Part print with two shaded views. Sizes in mm from the minimum x, y, z corner. A direction names the side the tool comes from. Round coordinates to 2 decimals unless told otherwise and drop trailing zeros. Order: outer loops, then holes, each group sorted by start corner. A loop starts at its lowest first (then second) coordinate and runs counter-clockwise, first axis right, second up. Notation, with made-up numbers: (85, 15.25) -> (133, 15.25) arc R13 ccw to (133, 29.25) -> close; hole circle Ø8 at (-14.5, 45.5). An arc over 180 degrees is marked (long way). Answer as a JSON object with one key per item and string values.
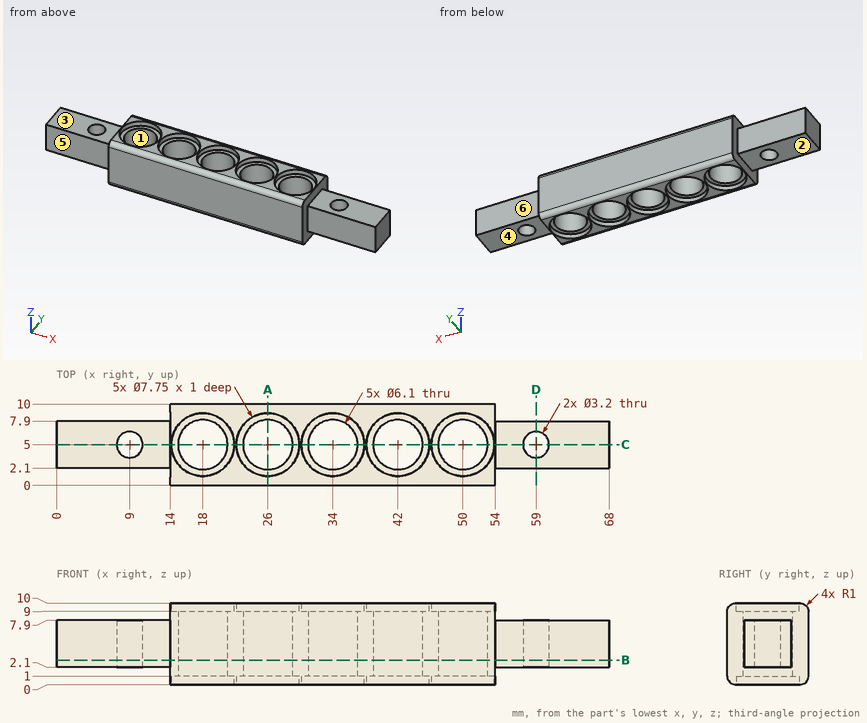
1) Cut at B-B, the plane z = 3. Give the cut face in (x, y), plus the area to 3 significant figures.
Checked values:
{"outline": "(0, 2.1) -> (14, 2.1) -> (14, 0) -> (54, 0) -> (54, 2.1) -> (68, 2.1) -> (68, 7.9) -> (54, 7.9) -> (54, 10) -> (14, 10) -> (14, 7.9) -> (0, 7.9) -> close; hole circle Ø3.2 at (9, 5); hole circle Ø6.1 at (18, 5); hole circle Ø6.1 at (26, 5); hole circle Ø6.1 at (34, 5); hole circle Ø6.1 at (42, 5); hole circle Ø6.1 at (50, 5); hole circle Ø3.2 at (59, 5)", "area": "400 mm²"}
2) Pull direction X, two halves, no side cores. Call the marked faces 1 and 2: pulls with the +X half, pulls with the -X half, needs draft (parallel to the pull), parting line crosses it, or undercut.
Checked values:
{"face 1": "undercut", "face 2": "needs draft"}
3) Cut at A-A, the plane x = 26. Give the cut face in (y, z) (3 decimals).
Checked values:
{"outline": "(0, 1) arc R1 ccw to (1, 0) -> (1.125, 0) -> (1.125, 1) -> (1.95, 1) -> (1.95, 9) -> (1.125, 9) -> (1.125, 10) -> (1, 10) arc R1 ccw to (0, 9) -> close; (8.05, 1) -> (8.875, 1) -> (8.875, 0) -> (9, 0) arc R1 ccw to (10, 1) -> (10, 9) arc R1 ccw to (9, 10) -> (8.875, 10) -> (8.875, 9) -> (8.05, 9) -> close"}
4) Flat gauge pins, fed straight in: pin 1 Ø2.5 at (x, y) = (43, 6) entering from +Z; pin 2 Ø1 at (y, z) = (7, 1.5) entering from +X; pin 3 Ø4.5 at (x, z) = (64.5, 5.5) entering from +Y; pin 4 Ø1.5 at (x, y) = (49, 2.5) entering from -Z. Where does each tip first touch, or does it go through?
Checked values:
{"pin 1": "passes through", "pin 2": "stops at x = 54", "pin 3": "stops at y = 7.9", "pin 4": "stops at z = 1"}
5) Probe L1, parallel to X at y = 6.5, z = 2; L2, parallel to X at y = 7.75, z = 2; L3, parallel to Y at x = 30.5, z = 0.5. List the from-to ranges inside material, lowest first. Write a range as from..to.
Checked values:
{"L1": "x = 14..15.34, 20.66..23.34, 28.66..31.34, 36.66..39.34, 44.66..47.34, 52.66..54", "L2": "x = 14..16.68, 19.32..24.68, 27.32..32.68, 35.32..40.68, 43.32..48.68, 51.32..54", "L3": "y = 0.13..3.34, 6.66..9.87"}
6) Which spindle directions (+Z, -Z, +X, -X, +Y, -Y) get a long thin tool onto all of the face, cutting with end or side? Do the marked faces 3, 4, 5 and 6. Say none if no direction does.
Checked values:
{"face 3": "+Z, -X, +Y, -Y", "face 4": "-Z, +X, +Y, -Y", "face 5": "+Z, -Z, -X, -Y", "face 6": "+Z, -Z, +X, +Y"}
7) Cut at D-D, the plane x = 59. Give the cut face in (y, z).
Checked values:
{"outline": "(2.1, 2.1) -> (3.4, 2.1) -> (3.4, 7.9) -> (2.1, 7.9) -> close; (6.6, 2.1) -> (7.9, 2.1) -> (7.9, 7.9) -> (6.6, 7.9) -> close"}
8) Cut at C-C, the plane y = 5. Count the separate pieces of the cut face and the enclosed holes in it, plus the area to 3 significant figures.
Checked values:
{"separate pieces": "8", "enclosed holes": "0", "area": "204 mm²"}
